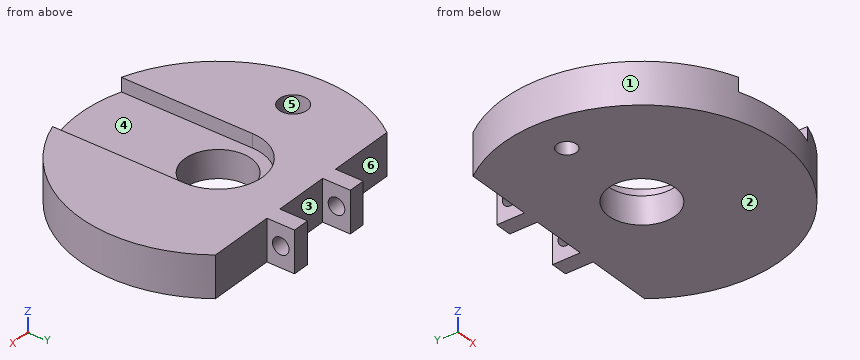
from build123d import *

# Parameters (mm, degrees)
ESTRUSIONE_ESTRUSIONE1_DEPTH                         = 15
TAGLIO_ESTRUSIONE1_DEPTH                             = 5
FORO_6_0_6_1_D                                       = 6
FORO_LAMATO_PER_BULLONE_M5_A_TESTA_ESAGO_D           = 7
FORO_LAMATO_PER_BULLONE_M5_A_TESTA_ESAGO_CBORE_D     = 10
FORO_LAMATO_PER_BULLONE_M5_A_TESTA_ESAGO_CBORE_DEPTH = 10
FORO_24_0_24_1_D                                     = 24


with BuildPart() as part:
    # Schizzo1 → Estrusione-Estrusione1 (new body)
    with BuildSketch(Plane.XY):
        with BuildLine():
            Line((-40, 30), (-16, 30))
            Line((-16, 30), (-16, 40))
            Line((-16, 40), (-10, 40))
            Line((-10, 40), (-10, 30))
            Line((-10, 30), (10, 30))
            Line((10, 30), (10, 40))
            Line((10, 40), (16, 40))
            Line((16, 40), (16, 30))
            Line((16, 30), (40, 30))
            ThreePointArc((40, 30), (0, -50), (-40, 30))
        make_face()
    extrude(amount=ESTRUSIONE_ESTRUSIONE1_DEPTH)

    # Schizzo2 → Taglio-Estrusione1 (cut)
    with BuildSketch(Plane.XY.offset(15)):
        with BuildLine():
            Line((-16.05, 0), (-16.05, -50))
            Line((-16.05, -50), (16.05, -50))
            Line((16.05, -50), (16.05, 0))
            ThreePointArc((16.05, 0), (0, 16.05), (-16.05, 0))
        make_face()
    extrude(amount=-TAGLIO_ESTRUSIONE1_DEPTH, mode=Mode.SUBTRACT)

    # Foro Ø6.0 (6)-1 (through all)
    with Locations(Plane.ZY.offset(16)):
        with Locations((7.5, 35)):
            Hole(FORO_6_0_6_1_D / 2)

    # Foro lamato per Bullone M5 a testa esagonale-1 (through all)
    with Locations(Plane.XY.offset(15)):
        with Locations((-35, 0)):
            CounterBoreHole(FORO_LAMATO_PER_BULLONE_M5_A_TESTA_ESAGO_D / 2, FORO_LAMATO_PER_BULLONE_M5_A_TESTA_ESAGO_CBORE_D / 2, FORO_LAMATO_PER_BULLONE_M5_A_TESTA_ESAGO_CBORE_DEPTH)

    # Foro Ø24.0 (24)-1 (through all)
    with Locations(Plane.XY.offset(10)):
        with Locations((0, 0)):
            Hole(FORO_24_0_24_1_D / 2)


solid = part.part
CAD build for the part. Positions are in the model's coordinates, mm. Face numbers are marked on the shaded views. A direction names the side the tool comes from. Round coordinates to 2 decimals unless told otherwise and drop trailing zeros. Write each loop counter-clockwise with the first axis right and the second up, starting at its lowest first coordinate (ties: lowest second). Pieces come first, ordered by that corner, then holes. Notation, with made-up numbers: M 60.25,18 L 103.25,18 A17 cw 103.25,23 Z; hole C 89.25,86 d6. An arc over 180 degrees is marked long. Put each result on its own line as item: value. Start each with the question number.
1) Saw through at C-C, the plane x = 0. Write the cut outline in (y, z), and give its area (3 significant figures).
2) 3-axis set-ups, long thin cutter, end or side, ignore diameter. For the marked faces 4, 5 and 6: which of +Z, -Z, +X, -X, +Y, -Y reach the whole face in a straight line?
3) Pull direction X, two halves, no side cores. Call the marked faces 1, 2 and 3: pulls with the +X half, pulls with the -X half, needs draft (parallel to the pull), parting line crosses it, or undercut.
4) Saw through at A-A, the plane z = 7.5. Write the cut outline in (x, y).
5) Pin check, flat tips, straight feed: pin 1 Ø6 at (y, z) = (26.5, 12) entering from -X; pin 2 Ø3 at (y, z) = (34, 9.5) entering from +X; pin 3 Ø3 at (y, z) = (26.5, 7.5) entering from -X; pin 4 Ø8 at (x, y) = (6.5, -1) entering from +Z. Stop position of each tip, or through.
6) Saw through at D-D, the plane y = 8. Write the cut outline in (x, z), and give its area (3 significant figures).
7) Drill centre lines: probe 1 along X at (y, z) = (34, 2); probe 2 along X at (y, z) = (-8.5, 13.5); probe 3 along Z at (x, y) = (14, 36.5). Where is each one in solid material? Low to high. Write a range as [from, to].
8) Saw through at B-B, the plane y = 35. Write the cut outline in (x, z).
Resolved:
1. outline: M -50,0 L -12,0 L -12,10 L -50,10 Z; M 12,0 L 30,0 L 30,15 L 16.05,15 L 16.05,10 L 12,10 Z
1. area: 630 mm²
2. face 4: +Z, -Y
2. face 5: +Z
2. face 6: +Z, -Z, -X, +Y
3. face 1: parting line crosses it
3. face 2: needs draft
3. face 3: undercut
4. outline: M -40,30 A50 ccw long 40,30 L 16,30 L 16,32 L 10,32 L 10,30 L -10,30 L -10,32 L -16,32 L -16,30 Z; M -16,38 L -10,38 L -10,40 L -16,40 Z; M 10,38 L 16,38 L 16,40 L 10,40 Z; hole C -35,0 d10; hole C 0,0 d24
5. pin 1: x = -44.13
5. pin 2: x = 16
5. pin 3: x = -43.3
5. pin 4: through
6. outline: M -49.36,0 L -8.94,0 L -8.94,10 L -13.91,10 L -13.91,15 L -49.36,15 Z; M 8.94,0 L 49.36,0 L 49.36,15 L 13.91,15 L 13.91,10 L 8.94,10 Z
6. area: 1,160 mm²
7. probe 1: [-16, -10], [10, 16]
7. probe 2: [-49.27, -16.05], [16.05, 49.27]
7. probe 3: [0, 4.9], [10.1, 15]
8. outline: M -16,0 L -10,0 L -10,4.5 L -16,4.5 Z; M -16,10.5 L -10,10.5 L -10,15 L -16,15 Z; M 10,0 L 16,0 L 16,4.5 L 10,4.5 Z; M 10,10.5 L 16,10.5 L 16,15 L 10,15 Z
